Model file for the job. Use its own axes, mm. A direction names the side the tool comes from. Round coordinates to 2 decimals unless told otherwise and drop trailing zeros. Return JSON: item names as keys, results as strings. Group by question number.
Item 1: Which spindle directions (+Z, -Z, +X, -X, +Y, -Y) get a long thin tool onto all of the face, cutting with end or side? Do faces 3 (the face through (10.44, -17.65, -7.66)), 4 (the face through (10.32, -6.97, 1.55)), 5 (the face through (6.148, 1.4, 1.4)). Say none if no direction does.
Item 2: Slice it at A-A on x = 4. Give the number of separate pieces and of enclosed holes in the cut face, then the cut area to 3 significant figures.
Item 3: Pull direction Z, two halves, no side cores. Call faces 1 (the face through (6.11, 9.49, 0.13)), 2 (the face through (5.982, 22.804, 2.994)): pulls with the +Z half, pulls with the -Z half, needs draft (parallel to the pull), parting line crosses it, or undercut.
Item 4: Probe line 1 along Y through (x, z) = (1, 0); line 2 along Y through (x, z) = (16.2, 0); line 3 along Y through (x, z) = (11, -0.5). List the from-to ranges inside material, lowest first.
Item 5: Pin check, flat tips, straight feed: pin 1 Ø6 at (x, y) = (7.5, -16) entering from -Z; pin 2 Ø1.5 at (x, z) = (15, 0.5) entering from -Y; pin 3 Ø12.5 at (y, z) = (-9, 10.5) entering from +X. Stop position of each tip, or through.
from build123d import *

# Parameters (mm, degrees)
SKETCH2_R               = 3.75
CUT_EXTRUDE2_DEPTH      = 19.15
CUT_EXTRUDE2_DEPTH_BACK = 6.85
CUT_EXTRUDE3_REACH      = 19.9
SKETCH3_R               = 1
CUT_EXTRUDE4_DEPTH      = 6.148


with BuildPart() as part:
    # Sketch1 → Revolve1 (revolve)
    with BuildSketch(Plane(origin=(0, 0, 0), x_dir=(1, 0, 0), z_dir=(0, 1, 0))):
        with BuildLine():
            Line((8.55, 1.6383), (8.55, 7.1383))
            Line((8.55, 7.1383), (12.05, 7.1383))
            Line((12.05, 7.1383), (12.05, 11.5))
            Line((12.05, 11.5), (14.05, 11.5))
            ThreePointArc((14.05, 11.5), (14.583745157, 15.635516896), (16.15, 19.5))
            Line((16.15, 19.5), (16.4, 19.5))
            Line((16.4, 19.5), (16.4, 21))
            Line((16.4, 21), (18.15, 21))
            Line((18.15, 21), (18.15, 23))
            Line((18.15, 23), (-5.85, 23))
            Line((-5.85, 23), (-5.85, 21))
            Line((-5.85, 21), (-4.35, 19.5))
            Line((-4.35, 19.5), (7, 19.5))
            Line((7, 19.5), (7, 9.75))
            Line((7, 9.75), (0, 9.75))
            Line((0, 9.75), (0, 1.6383))
            Line((0, 1.6383), (8.55, 1.6383))
        make_face()
    revolve(axis=Axis((0, 0, 0), (1, 0, 0)))

    # Sketch2 → Cut-Extrude2 (cut, two sides)
    with BuildSketch(Plane(origin=(0, 0, 0), x_dir=(0, 0, -1), z_dir=(1, 0, 0))) as cut_extrude2_sk:
        with Locations((-5.931593202, 14.320132754)):
            Circle(SKETCH2_R)
        with Locations((5.931593202, 14.320132754)):
            Circle(SKETCH2_R)
        with Locations((14.320132754, 5.931593202)):
            Circle(SKETCH2_R)
        with Locations((14.320132754, -5.931593202)):
            Circle(SKETCH2_R)
        with Locations((5.931593202, -14.320132754)):
            Circle(SKETCH2_R)
        with Locations((-5.931593202, -14.320132754)):
            Circle(SKETCH2_R)
        with Locations((-14.320132754, -5.931593202)):
            Circle(SKETCH2_R)
        with Locations((-14.320132754, 5.931593202)):
            Circle(SKETCH2_R)
    extrude(amount=CUT_EXTRUDE2_DEPTH, mode=Mode.SUBTRACT)
    extrude(cut_extrude2_sk.sketch, amount=-CUT_EXTRUDE2_DEPTH_BACK, mode=Mode.SUBTRACT)

    # Sketch3 → Cut-Extrude3 (cut, up to next)
    with BuildSketch(Plane(origin=(12.05, 0, 0), x_dir=(0, 0, -1), z_dir=(1, 0, 0)), mode=Mode.PRIVATE) as cut_extrude3_sk1:
        with Locations((0, 8.5)):
            Circle(SKETCH3_R)
    cut_extrude3_tool1 = extrude(cut_extrude3_sk1.sketch, amount=-CUT_EXTRUDE3_REACH, mode=Mode.PRIVATE) & part.part
    add(cut_extrude3_tool1.solids().sort_by_distance((12.05, 8.5, 0))[0], mode=Mode.SUBTRACT)
    # Sketch3 → Cut-Extrude3 (cut, up to next)
    with BuildSketch(Plane(origin=(12.05, 0, 0), x_dir=(0, 0, -1), z_dir=(1, 0, 0)), mode=Mode.PRIVATE) as cut_extrude3_sk2:
        with Locations((8.083980389, 2.626644452)):
            Circle(SKETCH3_R)
    cut_extrude3_tool2 = extrude(cut_extrude3_sk2.sketch, amount=-CUT_EXTRUDE3_REACH, mode=Mode.PRIVATE) & part.part
    add(cut_extrude3_tool2.solids().sort_by_distance((12.05, 2.626644, -8.08398))[0], mode=Mode.SUBTRACT)
    # Sketch3 → Cut-Extrude3 (cut, up to next)
    with BuildSketch(Plane(origin=(12.05, 0, 0), x_dir=(0, 0, -1), z_dir=(1, 0, 0)), mode=Mode.PRIVATE) as cut_extrude3_sk3:
        with Locations((4.996174644, -6.876644452)):
            Circle(SKETCH3_R)
    cut_extrude3_tool3 = extrude(cut_extrude3_sk3.sketch, amount=-CUT_EXTRUDE3_REACH, mode=Mode.PRIVATE) & part.part
    add(cut_extrude3_tool3.solids().sort_by_distance((12.05, -6.876644, -4.996175))[0], mode=Mode.SUBTRACT)
    # Sketch3 → Cut-Extrude3 (cut, up to next)
    with BuildSketch(Plane(origin=(12.05, 0, 0), x_dir=(0, 0, -1), z_dir=(1, 0, 0)), mode=Mode.PRIVATE) as cut_extrude3_sk4:
        with Locations((-4.996174644, -6.876644452)):
            Circle(SKETCH3_R)
    cut_extrude3_tool4 = extrude(cut_extrude3_sk4.sketch, amount=-CUT_EXTRUDE3_REACH, mode=Mode.PRIVATE) & part.part
    add(cut_extrude3_tool4.solids().sort_by_distance((12.05, -6.876644, 4.996175))[0], mode=Mode.SUBTRACT)
    # Sketch3 → Cut-Extrude3 (cut, up to next)
    with BuildSketch(Plane(origin=(12.05, 0, 0), x_dir=(0, 0, -1), z_dir=(1, 0, 0)), mode=Mode.PRIVATE) as cut_extrude3_sk5:
        with Locations((-8.083980389, 2.626644452)):
            Circle(SKETCH3_R)
    cut_extrude3_tool5 = extrude(cut_extrude3_sk5.sketch, amount=-CUT_EXTRUDE3_REACH, mode=Mode.PRIVATE) & part.part
    add(cut_extrude3_tool5.solids().sort_by_distance((12.05, 2.626644, 8.08398))[0], mode=Mode.SUBTRACT)

    # Sketch4 → Cut-Extrude4 (cut)
    with BuildSketch(Plane.ZY):
        Polygon((6.92820323, 0), (3.464101615, 6), (-3.464101615, 6), (-6.92820323, 0), (-3.464101615, -6), (3.464101615, -6), align=None)
    extrude(amount=-CUT_EXTRUDE4_DEPTH, mode=Mode.SUBTRACT)


solid = part.part
Output values:
{
 "1": {"face 3": "+X, -X", "face 4": "+X", "face 5": "-X"},
 "2": {"separate pieces": "2", "enclosed holes": "7", "area": "626 mm²"},
 "3": {"face 1": "undercut", "face 2": "parting line crosses it"},
 "4": {"line 1": "-23 to -19.5, -9.75 to -6, 6 to 7.5, 9.5 to 9.75, 19.5 to 23", "line 2": "-23 to -19.5, 19.5 to 23", "line 3": "-22.99 to -7.12, 7.12 to 7.63, 9.37 to 22.99"},
 "5": {"pin 1": "z = -18.97", "pin 2": "y = -23", "pin 3": "x = 16.4"}
}
